Can you work these out from the drawing? Everything is in mm from the part's minimum corner. A direction names the side the tool comes from. Coordinates: 2 decimals unless noted, no trailing zeros. Order: outer loops, then holes, each group sorted by start corner. A loop starts at its lowest first (then second) coordinate and runs counter-clockwise, first axis right, second up. Notation, with made-up numbers: (0.25, 33.25) -> (42.25, 33.25) arc R11 cw to (42.25, 53.25) -> close; hole circle Ø1 at (-5, 62). An arc over 180 degrees is marked (long way). Use a Markdown table: item, result. Add a question column.
1) Will these pins go through, and if not, where does the flat tip stop? pin 1 Ø2 at (x, z) = (20.5, 26.5) entering from -Y; pin 2 Ø8 at (x, z) = (11, 30.5) entering from +Y; pin 3 Ø3.5 at (y, z) = (14, 4) entering from -X; pin 4 Ø1.7 at (x, z) = (6.5, 7.5) entering from -Y.
2) If we section it at B-B (y = 13.9): Write out the boundary of the cut face in (x, z).
3) If we section it at D-D (z = 27.5): Write out the boundary of the cut face in (x, y).
4) If we section it at C-C (z = 6): Write out the boundary of the cut face in (x, y), plus the area to 3 significant figures.
5) If we section it at A-A (x = 13.9): Write out the boundary of the cut face in (y, z).
6) If I drill on L1, parallel to Z at x = 7.75, y = 25.5; L2, parallel to Z at x = 10.25, y = 13.5; L3, parallel to X at y = 11.5, z = 25, over which ranges is the centre line in solid material (lowest first)? Write a range as [from, to].
7) Which directions (+Z, -Z, +X, -X, +Y, -Y) give clear straight access to the entire face, cutting with the end or side of a thin tool? Please do the marked faces 1, 2 and 3.
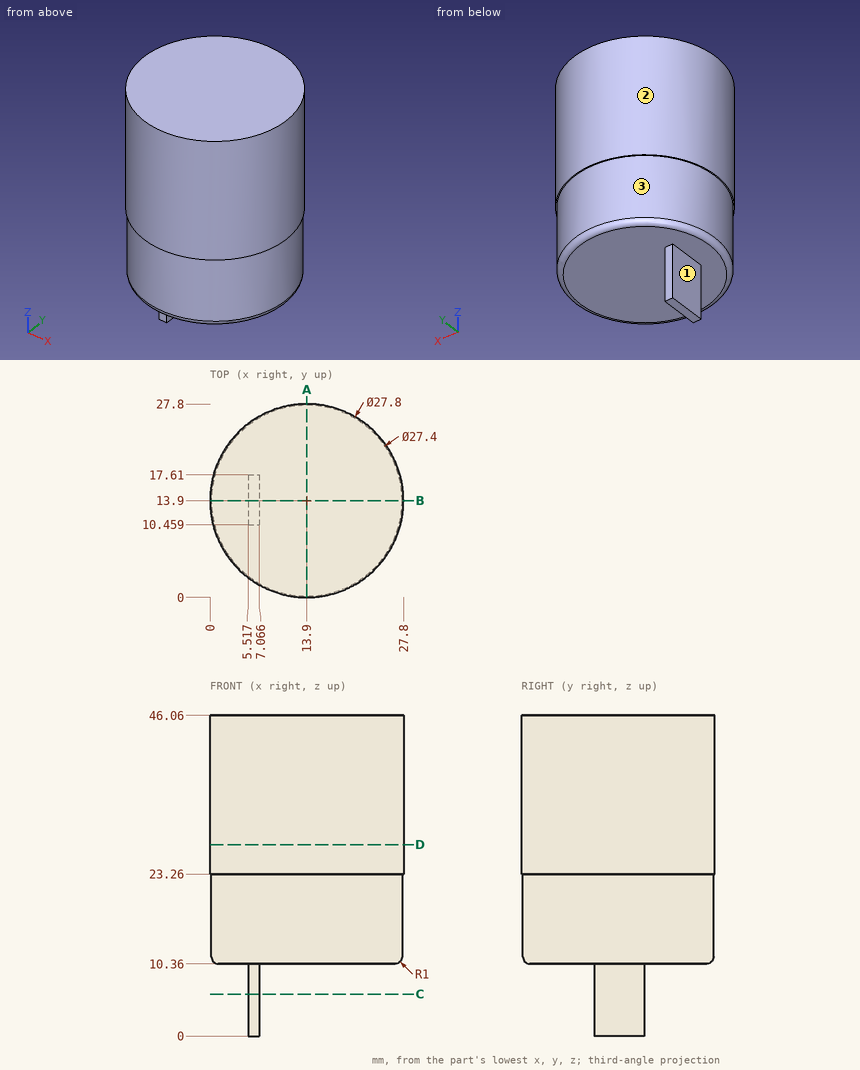
Answer sheet:
| question | item | result |
|---|---|---|
| 1 | pin 1 | y = 1.18 |
| 1 | pin 2 | y = 27.8 |
| 1 | pin 3 | x = 5.52 |
| 1 | pin 4 | y = 10.46 |
| 2 | outline | (0, 23.26) -> (0.2, 23.26) -> (0.2, 11.36) arc R1 ccw to (1.2, 10.36) -> (5.52, 10.36) -> (5.52, 0) -> (7.07, 0) -> (7.07, 10.36) -> (26.6, 10.36) arc R1 ccw to (27.6, 11.36) -> (27.6, 23.26) -> (27.8, 23.26) -> (27.8, 46.06) -> (0, 46.06) -> close |
| 3 | outline | circle Ø27.8 at (13.9, 13.9) |
| 4 | outline | (5.52, 10.46) -> (7.07, 10.46) -> (7.07, 17.61) -> (5.52, 17.61) -> close |
| 4 | area | 11.1 mm2 |
| 5 | outline | (0, 23.26) -> (0.2, 23.26) -> (0.2, 11.36) arc R1 ccw to (1.2, 10.36) -> (26.6, 10.36) arc R1 ccw to (27.6, 11.36) -> (27.6, 23.26) -> (27.8, 23.26) -> (27.8, 46.06) -> (0, 46.06) -> close |
| 6 | L1 | [10.46, 46.06] |
| 6 | L2 | [10.36, 46.06] |
| 6 | L3 | [0.21, 27.59] |
| 7 | face 1 | -Z, -X, +Y, -Y |
| 7 | face 2 | +Z, -Z |
| 7 | face 3 | -Z |
